Check sheet for the modelled part. Datum: model origin and axes. Units: mm. Round coordinates to 2 decimals unless told otherwise and drop trailing zeros. Order: outer loops, then holes, each group sorted by start corner. A loop starts at its lowest first (then second) coordinate and runs counter-clockwise, first axis right, second up. Notation, with made-up numbers: (7, 14) -> (13, 14) arc R16 cw to (13, 20) -> close; hole circle Ø9 at (18.25, -13.75). An arc over 180 degrees is marked (long way). Answer in a Markdown table with one row per item.
from build123d import *

# Parameters (mm, degrees)
SKETCH1_W             = 40.64
SKETCH1_H             = 2.54
BOSS_EXTRUDE1_DEPTH   = 2.54
F_1_0MM_DOWEL_HOLE1_D = 1.02
LPATTERN1_COUNT       = 16
LPATTERN1_PITCH       = 2.54


with BuildPart() as part:
    # Sketch1 → Boss-Extrude1 (new body)
    with BuildSketch(Plane(origin=(0, 0, 0), x_dir=(0, 0, -1), z_dir=(1, 0, 0))):
        Rectangle(SKETCH1_W, SKETCH1_H)
    extrude(amount=BOSS_EXTRUDE1_DEPTH)

    # Ø1.0mm Dowel Hole1 (through all)
    with Locations(Plane(origin=(1.27, 1.27, 19.05), x_dir=(0, 0, 1), z_dir=(0, 1, 0))):
        with Locations((0, 0)):
            f_1_0mm_dowel_hole1 = Hole(F_1_0MM_DOWEL_HOLE1_D / 2)

    # LPattern1: Ø1.0mm Dowel Hole1 ×16
    with Locations(*[(0, 0, -i * LPATTERN1_PITCH) for i in range(1, LPATTERN1_COUNT)]):
        add(f_1_0mm_dowel_hole1, mode=Mode.SUBTRACT)


solid = part.part
Item 1: Cross-section at B-B (y = 0.4). State how many separate pieces and enclosed holes the cut face has, and give its area (3 significant figures).
Result sheet:
| item | result |
|---|---|
| separate pieces | 1 |
| enclosed holes | 16 |
| area | 90.2 mm^2 |
Item 2: Cross-section at A-A (z = -16.51). Record the boundary of the cut face in (x, y), and give its area (3 significant figures).
Result sheet:
| item | result |
|---|---|
| outline | (0, -1.27) -> (0.76, -1.27) -> (0.76, 1.27) -> (0, 1.27) -> close; (1.78, -1.27) -> (2.54, -1.27) -> (2.54, 1.27) -> (1.78, 1.27) -> close |
| area | 3.86 mm^2 |
Item 3: Mould release check, pull along X, two halves, no side actions. Record for faces 1 (the flat face through (2.54, 0, 0)), 2 (the flat face through (1, -1.27, 0)), 3 (the cylindrical face through (1.423, -0.018, -16.996)): pulls with the +X half, pulls with the -X half, needs draft (parallel to the pull), parting line crosses it, or undercut.
Result sheet:
| item | result |
|---|---|
| face 1 | pulls with the +X half |
| face 2 | needs draft |
| face 3 | undercut |
Item 4: Scan lines: line 1 (X direction, y = 0.2, z = -11.43); line 2 (X direction, y = 1.15, z = -11). Record each from-to range of solid material in increasing order. Write a range as [from, to].
Result sheet:
| item | result |
|---|---|
| line 1 | x = [0, 0.76], [1.78, 2.54] |
| line 2 | x = [0, 1], [1.54, 2.54] |
